Read the model definition and answer for the solid it produces. Units are mm, in the model's axes. A direction names the side the tool comes from. Round coordinates to 2 decimals unless told otherwise and drop trailing zeros. Write each loop counter-clockwise with the first axis right and the second up, starting at its lowest first coordinate (ties: lowest second). Pieces come first, ordered by that corner, then holes.
from build123d import *

# Parameters (mm, degrees)
BOSS_EXTRUDE1_DEPTH = 17
BOSS_EXTRUDE2_DEPTH = 10
BOSS_EXTRUDE3_DEPTH = 29
SKETCH6_R           = 4
BOSS_EXTRUDE4_DEPTH = 8
BOSS_EXTRUDE5_DEPTH = 26
SKETCH11_R          = 2.5
BOSS_EXTRUDE6_DEPTH = 9
BOSS_EXTRUDE8_START = 3
BOSS_EXTRUDE8_DEPTH = 3
CUT_EXTRUDE1_DEPTH  = 3
BOSS_EXTRUDE7_START = 2
SKETCH12_R          = 5
BOSS_EXTRUDE7_DEPTH = 5
BOSS_EXTRUDE7_TAPER = -45
SKETCH10_W          = 10
SKETCH10_H          = 17
CUT_EXTRUDE2_DEPTH  = 9.2
CUT_EXTRUDE3_START  = -13.5
SKETCH14_W          = 25
SKETCH14_H          = 5
CUT_EXTRUDE3_DEPTH  = 57.929042368
SKETCH15_R          = 2.5
CUT_EXTRUDE4_DEPTH  = 8
SKETCH16_R          = 1.5
CUT_EXTRUDE5_DEPTH  = 6
SKETCH17_R          = 2.5
CUT_EXTRUDE6_DEPTH  = 21.5
FILLET1_R           = 6


with BuildPart() as part:
    # Sketch1 → Boss-Extrude1 (new body)
    with BuildSketch(Plane(origin=(0, 0, 0), x_dir=(1, 0, 0), z_dir=(0, 1, 0))):
        with BuildLine():
            Line((-11, 16.5), (-36, 16.5))
            ThreePointArc((-36, 16.5), (-46.695268783, 8.071230378), (-41, -4.297958971))
            Line((-41, -4.297958971), (-41, -16.5))
            Line((-41, -16.5), (-11, -16.5))
            ThreePointArc((-11, -16.5), (-3.221825407, -13.278174593), (0, -5.5))
            Line((0, -5.5), (0, 5.5))
            ThreePointArc((0, 5.5), (-3.221825407, 13.278174593), (-11, 16.5))
        make_face()
    extrude(amount=BOSS_EXTRUDE1_DEPTH)

    # Sketch2 → Boss-Extrude2 (add)
    with BuildSketch(Plane(origin=(0, 17, 0), x_dir=(1, 0, 0), z_dir=(0, 1, 0))):
        with BuildLine():
            Line((-33.5, 16.5), (-32.471532465, 23.912304266))
            ThreePointArc((-32.471532465, 23.912304266), (-29.293357066, 26.492874655), (-26.5, 23.5))
            Line((-26.5, 23.5), (-26.5, 21.5))
            Line((-26.5, 21.5), (-20.5, 21.5))
            Line((-20.5, 21.5), (-20.5, 23.5))
            ThreePointArc((-20.5, 23.5), (-17.706642934, 26.492874655), (-14.528467535, 23.912304266))
            Line((-14.528467535, 23.912304266), (-13.5, 16.5))
            Line((-13.5, 16.5), (-33.5, 16.5))
        make_face()
    extrude(amount=-BOSS_EXTRUDE2_DEPTH)

    # Sketch5 → Boss-Extrude3 (add)
    with BuildSketch(Plane.XY.offset(44.5)):
        with BuildLine():
            Line((-11.5, 6.898979486), (-11.5, -2.898979486))
            ThreePointArc((-11.5, -2.898979486), (12.5, 2), (-11.5, 6.898979486))
        make_face()
    extrude(amount=-BOSS_EXTRUDE3_DEPTH)

    # Sketch6 → Boss-Extrude4 (add)
    with BuildSketch(Plane.ZY.offset(11.5)):
        with Locations(Location((36.5, 2, 0), (0, 0, 270))):
            Circle(SKETCH6_R)
    extrude(amount=BOSS_EXTRUDE4_DEPTH)

    # Sketch7 → Boss-Extrude5 (add)
    with BuildSketch(Plane(origin=(0, 17, 0), x_dir=(1, 0, 0), z_dir=(0, 1, 0))):
        with BuildLine():
            Line((-44, -8.5), (-35, -8.5))
            Line((-35, -8.5), (-35, -16.5))
            Line((-35, -16.5), (-44, -16.5))
            ThreePointArc((-44, -16.5), (-48, -12.5), (-44, -8.5))
        make_face()
    extrude(amount=-BOSS_EXTRUDE5_DEPTH)

    # Sketch11 → Boss-Extrude6 (add)
    with BuildSketch(Plane(origin=(0, 17, 0), x_dir=(1, 0, 0), z_dir=(0, 1, 0))):
        with Locations(Location((-23.5, 17.5, 0), (0, 0, 270))):
            Circle(SKETCH11_R)
        with Locations(Location((-34, -12.5, 0), (0, 0, 270))):
            Circle(SKETCH11_R)
        with Locations(Location((-13, -12.5, 0), (0, 0, 270))):
            Circle(SKETCH11_R)
    extrude(amount=BOSS_EXTRUDE6_DEPTH)

    # Sketch13 → Boss-Extrude8 (add)
    with BuildSketch(Plane.XZ.offset(BOSS_EXTRUDE8_START)):
        with BuildLine():
            Line((-11, -5.5), (0, -5.5))
            Line((0, -5.5), (0, 5.5))
            ThreePointArc((0, 5.5), (-18.778174593, 13.278174593), (-11, -5.5))
        make_face()
    extrude(amount=-BOSS_EXTRUDE8_DEPTH)

    # Sketch9 → Cut-Extrude1 (cut)
    with BuildSketch(Plane.XZ):
        with BuildLine():
            Line((-25, -16.5), (-25, -5.5))
            ThreePointArc((-25, -5.5), (-43.778174593, 2.278174593), (-36, -16.5))
            Line((-36, -16.5), (-25, -16.5))
        make_face()
    extrude(amount=-CUT_EXTRUDE1_DEPTH, mode=Mode.SUBTRACT)

    # Sketch12 → Boss-Extrude7 (add)
    with BuildSketch(Plane.XZ.offset(BOSS_EXTRUDE7_START)):
        with Locations((-36, -5.5)):
            Circle(SKETCH12_R)
    extrude(amount=-BOSS_EXTRUDE7_DEPTH, taper=BOSS_EXTRUDE7_TAPER)

    # Sketch10 → Cut-Extrude2 (cut)
    with BuildSketch(Plane.XY.offset(16.5)):
        with Locations((-43, 2)):
            Rectangle(SKETCH10_W, SKETCH10_H)
    extrude(amount=-CUT_EXTRUDE2_DEPTH, mode=Mode.SUBTRACT)

    # Sketch14 → Cut-Extrude3 (cut, through all)
    with BuildSketch(Plane(origin=(0, 0, 0), x_dir=(0, 0, -1), z_dir=(1, 0, 0)).offset(CUT_EXTRUDE3_START)):
        with Locations((14, 11.5)):
            Rectangle(SKETCH14_W, SKETCH14_H)
    extrude(amount=-CUT_EXTRUDE3_DEPTH, mode=Mode.SUBTRACT)

    # Sketch15 → Cut-Extrude4 (cut)
    with BuildSketch(Plane.ZY.offset(19.5)):
        with Locations(Location((36.5, 2, 0), (0, 0, 270))):
            Circle(SKETCH15_R)
    extrude(amount=-CUT_EXTRUDE4_DEPTH, mode=Mode.SUBTRACT)

    # Sketch16 → Cut-Extrude5 (cut)
    with BuildSketch(Plane(origin=(0, 26, 0), x_dir=(1, 0, 0), z_dir=(0, 1, 0))):
        with Locations(Location((-23.5, 17.5, 0), (0, 0, 270))):
            Circle(SKETCH16_R)
        with Locations(Location((-34, -12.5, 0), (0, 0, 270))):
            Circle(SKETCH16_R)
        with Locations(Location((-13, -12.5, 0), (0, 0, 270))):
            Circle(SKETCH16_R)
    extrude(amount=-CUT_EXTRUDE5_DEPTH, mode=Mode.SUBTRACT)

    # Sketch17 → Cut-Extrude6 (cut)
    with BuildSketch(Plane.XZ.offset(9)):
        with Locations(Location((-44, 12.5, 0), (0, 0, 270))):
            Circle(SKETCH17_R)
    extrude(amount=-CUT_EXTRUDE6_DEPTH, mode=Mode.SUBTRACT)

    # Fillet1
    # the kernel refuses this fillet: 6 mm, written as the material it adds along each edge
    with BuildSketch(Plane(origin=(-38, 10.5, 7.3), x_dir=(0, 0, 1), z_dir=(0, -1, 0))) as fillet1_piece_1_section:
        with BuildLine():
            CenterArc((5.196152423, 6), FILLET1_R, 210, 60)
            Line((0, 3), (0, 0))
            Line((0, 0), (5.196152423, 0))
        make_face()
    fillet1_piece_1 = extrude(amount=23.490381057, mode=Mode.PRIVATE)
    fillet1_piece_1 = split(fillet1_piece_1, bisect_by=Plane(origin=(-38.38283384, 5.25, 8.5), z_dir=(0, 0, 1)), keep=Keep.TOP, mode=Mode.PRIVATE)
    fillet1_piece_1 = split(fillet1_piece_1, bisect_by=Plane(origin=(-38.38283384, -9, 10.353353241), z_dir=(0, 1, 0)), keep=Keep.TOP, mode=Mode.PRIVATE)
    add(fillet1_piece_1)
    with BuildSketch(Plane(origin=(-38, 10.5, 7.3), x_dir=(0, 0, 1), z_dir=(0, -1, 0))) as fillet1_piece_2:
        with BuildLine():
            CenterArc((5.196152423, 6), FILLET1_R, 210, 60)
            Line((0, 3), (0, 0))
            Line((0, 0), (5.196152423, 0))
        make_face()
    extrude(amount=10.5)


solid = part.part
Q1. Section A-A (y = 23) is taken. Determine the outline of the cut face in (x, z), then the cut area to 3 significant figures.
Verdict:
outline: circle Ø5 at (-34, 12.5); circle Ø5 at (-23.5, -17.5); circle Ø5 at (-13, 12.5); hole circle Ø3 at (-34, 12.5); hole circle Ø3 at (-23.5, -17.5); hole circle Ø3 at (-13, 12.5)
area: 37.7 mm2
Q2. Section C-C (x = -3) is taken. Determine the outline of the cut face in (y, z), then the cut area to 3 significant figures.
Verdict:
outline: (-10.13, 15.5) - (14.13, 15.5) - (14.13, 44.5) - (-10.13, 44.5) - close; (-3, -5.5) - (0, -5.5) - (0, -13.05) - (17, -13.05) - (17, 13.05) - (-3, 13.05) - close
area: 1,200 mm2
Q3. Flat-ended cylindrical pins translate along their axes: pin 1 Ø2.5 at (y, z) = (1, 37.5) entering from -X; pin 2 Ø2 at (x, y) = (-35, 11.5) entering from -Z; pin 3 Ø1 at (y, z) = (-4.5, 17.5) entering from -X. Find the tip coordinate at first contact, or state that the pin passes through.
Verdict:
pin 1: stops at x = -19.5
pin 2: stops at z = -1.5
pin 3: stops at x = -10.97
Q4. Section B-B (z = 36.5) is taken. Determine the outline of the cut face in (x, y), then the cut area to 3 significant figures.
Verdict:
outline: (-19.5, -2) - (-11.5, -2) - (-11.5, -2.9) arc R12.5 ccw (long way) to (-11.5, 6.9) - (-11.5, 6) - (-19.5, 6) - (-19.5, 4.5) - (-11.5, 4.5) - (-11.5, -0.5) - (-19.5, -0.5) - close
area: 508 mm2
Q5. Straight lines are drawn through the part: probe 1 along X at (y, z) = (21.9, 12.5); probe 2 along Y at (x, z) = (-19.5, -3); probe 3 along Y at (x, z) = (-15, -2). For each, find the intervals that lie inside material, in ascending order.
Verdict:
probe 1: x = -36.5 to -35.5, -32.5 to -31.5, -15.5 to -14.5, -11.5 to -10.5
probe 2: y = 0 to 9, 14 to 17
probe 3: y = -3 to 9, 14 to 17
Q6. Section D-D (z = -17.5) is taken. Determine the outline of the cut face in (x, y).
Verdict:
outline: (-33.36, 7) - (-13.64, 7) - (-13.64, 9) - (-33.36, 9) - close; (-33.36, 14) - (-13.64, 14) - (-13.64, 17) - (-21, 17) - (-21, 26) - (-22, 26) - (-22, 20) - (-25, 20) - (-25, 26) - (-26, 26) - (-26, 17) - (-33.36, 17) - close
Q7. Determine the mould class of faces 6 (the flat face through (-35, 15, -16.5)), 7 (the cylindrical face through (-38.8, 2.1, 9.5)), 8 (the flat face through (-24, 8, -21.5)) for opening direction X: pulls with the +X half, pulls with the -X half, needs draft (parallel to the pull), parting line crosses it, or undercut.
Verdict:
face 6: needs draft
face 7: pulls with the -X half
face 8: undercut
Q8. Which of the six approach directions +Z, -Z, +X, -X, +Y, -Y give full straight-line access (tool end or side, diameter ignored) to faces 1 (the flat face through (-23, 20, -18)), 2 (the flat face through (-26.5, 16, -23)), 3 (the flat face through (-38, -5, 8.5)), 4 (the cylindrical face through (-46.44, 11.49, 13.04)), 5 (the flat face through (-30, 11, -1.5))?
Verdict:
face 1: +Y
face 2: -Z, +Y, -Y
face 3: -X, -Y
face 4: -Y
face 5: -Z, -X
